from build123d import *

# Parameters (mm, degrees)
SKETCH1_R                = 60
SKETCH1_R_2              = 12.5
BOSS_EXTRUDE2_DEPTH      = 30
SKETCH3_R                = 40
CUT_EXTRUDE3_DEPTH       = 10
SKETCH4_R                = 5.959098303
CUT_EXTRUDE4_DEPTH       = 21
SKETCH7_R                = 14
SKETCH7_R_2              = 12.5
BOSS_EXTRUDE6_DEPTH      = 2
BOSS_EXTRUDE6_DEPTH_BACK = 7


with BuildPart() as part:
    # Sketch1 → Boss-Extrude2 (new body)
    with BuildSketch(Plane.XY):
        Circle(SKETCH1_R)
        Circle(SKETCH1_R_2, mode=Mode.SUBTRACT)
    extrude(amount=BOSS_EXTRUDE2_DEPTH)

    # Sketch3 → Cut-Extrude3 (cut)
    with BuildSketch(Plane.XY.offset(30)):
        Circle(SKETCH3_R)
    cut_extrude3 = extrude(amount=-CUT_EXTRUDE3_DEPTH, mode=Mode.SUBTRACT)

    # Mirror6: Cut-Extrude3 across plane
    add(cut_extrude3.mirror(Plane.XY), mode=Mode.SUBTRACT)

    # Sketch4 → Cut-Extrude4 (cut, through all)
    with BuildSketch(Plane.XY.offset(20)):
        with Locations((0, 25)):
            Circle(SKETCH4_R)
        with Locations((23.776412907, 7.725424859)):
            Circle(SKETCH4_R)
        with Locations((14.694631307, -20.225424859)):
            Circle(SKETCH4_R)
        with Locations((-14.694631307, -20.225424859)):
            Circle(SKETCH4_R)
        with Locations((-23.776412907, 7.725424859)):
            Circle(SKETCH4_R)
    extrude(amount=-CUT_EXTRUDE4_DEPTH, mode=Mode.SUBTRACT)

    # Sketch6 → Cut-Revolve1 (revolve, cut)
    with BuildSketch(Plane(origin=(0, 0, 0), x_dir=(1, 0, 0), z_dir=(0, 1, 0))):
        Polygon((60, -3), (52.205771366, -7.5), (52.205771366, -22.5), (60, -27), align=None)
    revolve(axis=Axis((0, 0, 0), (0, 0, -1)), mode=Mode.SUBTRACT)

    # Sketch7 → Boss-Extrude6 (add, two sides)
    with BuildSketch(Plane.XY.offset(20)) as boss_extrude6_sk:
        Circle(SKETCH7_R)
        Circle(SKETCH7_R_2, mode=Mode.SUBTRACT)
    extrude(amount=BOSS_EXTRUDE6_DEPTH)
    extrude(boss_extrude6_sk.sketch, amount=-BOSS_EXTRUDE6_DEPTH_BACK)


solid = part.part
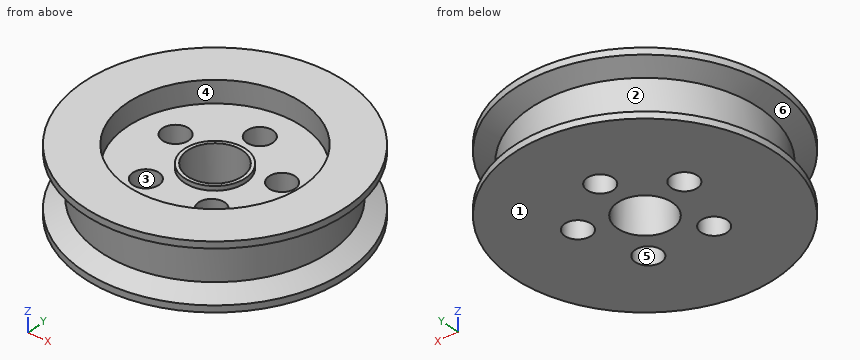
Geometry: final body of the model. Coordinates: model frame, mm. Face numbers are marked on the shaded views. A direction names the side the tool comes from. Round coordinates to 2 decimals unless told otherwise and drop trailing zeros. Order: outer loops, then holes, each group sorted by start corner. A loop starts at its lowest first (then second) coordinate and runs counter-clockwise, first axis right, second up.
Q1. Section D-D, the plane y = -24.5. Give the number of separate pieces and of enclosed holes in the cut face, and give its area (3 significant figures).
Result sheet:
separate pieces: 3
enclosed holes: 0
area: 1,980 mm2
Q2. Material intervals for probe 1 along Y at (x, z) = (0, 17.75); probe 2 along Y at (x, z) = (0, 4.25); probe 3 along Z at (x, y) = (1.5, -12.5), sorted ascending.
Result sheet:
probe 1: y = -52.21 to -12.5, 12.5 to 19.04, 30.96 to 52.21
probe 2: y = -57.83 to -12.5, 12.5 to 19.04, 30.96 to 57.83
probe 3: z = 0 to 22
Q3. Section A-A, the plane y = 0. Output: boundary loops of the cut face in (x, z).
Result sheet:
outline: (-60, 0) - (-12.5, 0) - (-12.5, 22) - (-14, 22) - (-14, 20) - (-40, 20) - (-40, 30) - (-60, 30) - (-60, 27) - (-52.21, 22.5) - (-52.21, 7.5) - (-60, 3) - close; (12.5, 0) - (60, 0) - (60, 3) - (52.21, 7.5) - (52.21, 22.5) - (60, 27) - (60, 30) - (40, 30) - (40, 20) - (14, 20) - (14, 22) - (12.5, 22) - close
Q4. Access query for the marked faces 4, 5 and 6. Directions: +Z, -Z, +X, -X, +Y, -Y. A direction counts if a zero-diameter tool reaches every point of the face in a straight line with its end or side. Return the directions, or none.
Result sheet:
face 4: +Z
face 5: +Z, -Z
face 6: none
Q5. Pin query (flat end, axial travel): pin 1 (13.5 mm diameter, centred on x = 23.78, y = 7.73, fed in from +Z); pin 2 (12 mm diameter, centred on y = 22.5, z = 19, fed in from +X); pin 3 (3 mm diameter, centred on y = 34.5, z = 5, fed in from +X). Return the tip coordinate at first contact, or that it passes through.
Result sheet:
pin 1: stops at z = 20
pin 2: stops at x = 52.14
pin 3: stops at x = 48.2
Q6. Section B-B, the plane x = 0. Output: boundary loops of the cut face in (y, z).
Result sheet:
outline: (-60, 0) - (-12.5, 0) - (-12.5, 22) - (-14, 22) - (-14, 20) - (-40, 20) - (-40, 30) - (-60, 30) - (-60, 27) - (-52.21, 22.5) - (-52.21, 7.5) - (-60, 3) - close; (12.5, 0) - (19.04, 0) - (19.04, 20) - (14, 20) - (14, 22) - (12.5, 22) - close; (30.96, 0) - (60, 0) - (60, 3) - (52.21, 7.5) - (52.21, 22.5) - (60, 27) - (60, 30) - (40, 30) - (40, 20) - (30.96, 20) - close
Q7. Section C-C, the plane z = 14. Output: boundary loops of the cut face in (x, y), and give its area (3 significant figures).
Result sheet:
outline: circle Ø104.41 at (0, 0); hole circle Ø11.92 at (-23.78, 7.73); hole circle Ø11.92 at (-14.69, -20.23); hole circle Ø25 at (0, 0); hole circle Ø11.92 at (0, 25); hole circle Ø11.92 at (14.69, -20.23); hole circle Ø11.92 at (23.78, 7.73)
area: 7,510 mm2
Q8. Mould query, pull axis Y, two halves, no side actions, for the marked faces 1, 2 and 3. Classes: released by +Y, released by -Y, zero draft, split by the parting line, or undercut.
Result sheet:
face 1: zero draft
face 2: split by the parting line
face 3: undercut
